Can you work these out from the model? Positions are in its coordinate system, mm. A direction names the side the tool comes from. Round coordinates to 2 decimals unless told otherwise and drop trailing zeros. Order: outer loops, then holes, each group sorted by start corner. A loop starts at its lowest first (then second) coordinate and runs counter-clockwise, first axis right, second up. Notation, with made-up numbers: (78.5, -39) -> (133.5, -39) arc R23 cw to (133.5, -23) -> close; hole circle Ø7 at (78, 20.5). An arc over 180 degrees is marked (long way). Use a Markdown table: item, result. Add a question column.
Q1. I need wall thicknesses on line 1 along Y through (x, z) = (-5.5, 0); line 2 along Z through (x, y) = (0.5, 4.5). Which ranges of each line are inside material? Lowest first, please. Write a range as [from, to].
Q2. We'd pull the mould along Y, two halves only. Please class faces 1 (the face through (0, 6, -1)), 2 (the face through (0, 4, 0)), 3 (the face through (-4.3, 0.1, -2.5)), 4 (the face through (-4, 0, 0)): +Y half, -Y half, draft (parallel to the pull), parting line (faces both ways), or undercut.
Q3. If we section it at A-A on x = 0: List the corners of the cut face in (y, z) for me, plus the area to 3 significant figures.
Q4. If we section it at D-D on z = -4.5: List the corners of the cut face in (x, y) for me, plus the area to 3 significant figures.
Q5. If we section it at B-B on y = 2: List the corners of the cut face in (x, z) for me.
Q6. I'm going to push flat-ended pins straight in: pin 1 Ø1.2 at (y, z) = (0, 0) entering from -X; pin 2 Ø8 at (x, y) = (4.5, -5) entering from -Z; pin 3 Ø1.8 at (x, z) = (0, 0) entering from -Y; pin 4 Ø3 at (x, y) = (-4.5, 4.5) entering from -Z. Where does each tip first touch, or does it pass through?
Q7. For faces 5 (the face through (-6, -1, 0)), 6 (the face through (0.1, -4.3, 2.5)), 7 (the face through (0, -1, -6)), which set-ups out of +Z, -Z, +X, -X, +Y, -Y let a thin tool reach every point of the face, with its end or its side?
```python
from build123d import *

# Parameters (mm, degrees)
SKETCH1_R           = 2.5
BASE_EXTRUDE_DEPTH  = 7
SKETCH2_R           = 2.5
BOSS_EXTRUDE3_DEPTH = 7
SKETCH3_R           = 2.5
BOSS_EXTRUDE4_DEPTH = 7
SKETCH8_R           = 1
CUT_EXTRUDE2_DEPTH  = 3
CIRPATTERN4_COUNT   = 4
CIRPATTERN5_COUNT   = 4


with BuildPart() as part:
    # Sketch1 → Base-Extrude (new, symmetric)
    with BuildSketch(Plane.XY):
        with Locations(Location((0, 0, 0), (0, 0, 225))):
            Circle(SKETCH1_R)
    extrude(amount=BASE_EXTRUDE_DEPTH, both=True)

    # Sketch2 → Boss-Extrude3 (add, symmetric)
    with BuildSketch(Plane(origin=(0, 0, 0), x_dir=(1, 0, 0), z_dir=(0, 1, 0))):
        with Locations(Location((0, 0, 0), (0, 0, 135))):
            Circle(SKETCH2_R)
    extrude(amount=BOSS_EXTRUDE3_DEPTH, both=True)

    # Sketch3 → Boss-Extrude4 (add, symmetric)
    with BuildSketch(Plane(origin=(0, 0, 0), x_dir=(0, 0, -1), z_dir=(1, 0, 0))):
        with Locations(Location((0, 0, 0), (0, 0, 225))):
            Circle(SKETCH3_R)
    extrude(amount=BOSS_EXTRUDE4_DEPTH, both=True)

    # Sketch8 → Cut-Extrude2 (cut)
    with BuildSketch(Plane(origin=(7, 0, 0), x_dir=(0, 0, -1), z_dir=(1, 0, 0))):
        Circle(SKETCH8_R)
    cut_extrude2 = extrude(amount=-CUT_EXTRUDE2_DEPTH, mode=Mode.SUBTRACT)

    # CirPattern4: Cut-Extrude2 ×4 about axis
    cirpattern4_axis = Axis((0, 0, 0), (0, 1, 0))
    for i in range(1, CIRPATTERN4_COUNT):
        add(cut_extrude2.rotate(cirpattern4_axis, i * 360 / CIRPATTERN4_COUNT), mode=Mode.SUBTRACT)

    # CirPattern5: Cut-Extrude2 ×4 about axis
    cirpattern5_axis = Axis((0, 0, 0), (0, 0, 1))
    for i in range(1, CIRPATTERN5_COUNT):
        add(cut_extrude2.rotate(cirpattern5_axis, i * 360 / CIRPATTERN5_COUNT), mode=Mode.SUBTRACT)


solid = part.part
```
Answer below:
| question | item | result |
|---|---|---|
| 1 | line 1 | [-2.5, -1], [1, 2.5] |
| 1 | line 2 | [-2.45, -0.87], [0.87, 2.45] |
| 2 | face 1 | draft |
| 2 | face 2 | +Y half |
| 2 | face 3 | parting line |
| 2 | face 4 | undercut |
| 3 | outline | (-7, -2.5) -> (-2.5, -2.5) -> (-2.5, -7) -> (-1, -7) -> (-1, -4) -> (1, -4) -> (1, -7) -> (2.5, -7) -> (2.5, -2.5) -> (7, -2.5) -> (7, -1) -> (4, -1) -> (4, 1) -> (7, 1) -> (7, 2.5) -> (2.5, 2.5) -> (2.5, 7) -> (1, 7) -> (1, 4) -> (-1, 4) -> (-1, 7) -> (-2.5, 7) -> (-2.5, 2.5) -> (-7, 2.5) -> (-7, 1) -> (-4, 1) -> (-4, -1) -> (-7, -1) -> close |
| 3 | area | 91.0 mm² |
| 4 | outline | circle Ø5 at (0, 0); hole circle Ø2 at (0, 0) |
| 4 | area | 16.5 mm² |
| 5 | outline | (-7, -1.5) -> (-2, -1.5) arc R2.5 ccw to (-1.5, -2) -> (-1.5, -7) -> (1.5, -7) -> (1.5, -2) arc R2.5 ccw to (2, -1.5) -> (7, -1.5) -> (7, 1.5) -> (2, 1.5) arc R2.5 ccw to (1.5, 2) -> (1.5, 7) -> (-1.5, 7) -> (-1.5, 2) arc R2.5 ccw to (-2, 1.5) -> (-7, 1.5) -> close |
| 6 | pin 1 | x = -4 |
| 6 | pin 2 | z = -2.45 |
| 6 | pin 3 | y = -4 |
| 6 | pin 4 | through |
| 7 | face 5 | -X |
| 7 | face 6 | -Y |
| 7 | face 7 | -Z |
